```python
from build123d import *

# Parameters (mm, degrees)
F0_W = 76.971642673
F0_H = 95.2017754316


# Not quite as in the source:
# - a feature names something its author has since deleted; it is built from what else it names
# - the program builds the solid bodies; features that only make, move or delete a surface that nothing else refers to are left out


with BuildPart() as f2:
    # F2: sweep along a path in F1
    with BuildLine(Plane.XY) as f2_path:
        ThreePointArc((0, 0), (13.4369935077, -32.3954640503), (39.643291384, -55.703163147))
    # F0 (on Front) → F2 (sweep)
    with BuildSketch(Plane.XZ):
        Rectangle(F0_W, F0_H)
    sweep(path=f2_path.line)

    # F3: sweep along a path in F1
    with BuildLine(Plane.XY) as f3_path:
        ThreePointArc((-40.5113920569, -54.2563311756), (-14.8539477386, -31.1614707896), (0, 0))
    # F0 (on Front) → F3 (sweep)
    with BuildSketch(Plane.XZ):
        Rectangle(F0_W, F0_H)
    sweep(path=f3_path.line)


solid = f2.part
```
Model file for the job. Use its own axes, mm. A direction names the side the tool comes from. Coordinates: 2 decimals unless noted, no trailing zeros. Loops run counter-clockwise (first coordinate to the right, second up) from the corner with the lowest first, then second, coordinate; pieces in that order, holes last. Notation, with made-up numbers: M 7,-24 L 37,-24 A25 ccw 37,-4 Z; hole C -16,-35.5 d9. An arc over 180 degrees is marked long. Use CSV: the item, a comma, the result in double quotes. Start each with the question number.
1. Flat gauge pin, fed straight in: pin 1 (1.5 mm diameter, centred on y = -10.5, z = -1.5, fed in from +X). Where does the tip first touch, or does it go through?
2. Probe probe 1 along X at (y, z) = (-79, 15.5); probe 2 along X at (y, z) = (-77, -9); probe 3 along X at (y, z) = (-66, 1). List the from-to ranges inside material, lowest first. Write a range as [from, to].
3. Band-saw the part on B-B, the plane z = -1. List the corners of the cut face in (x, y).
4. Band-saw the part on C-C, the plane x = 5.5. List the corners of the cut face in (y, z), then the cut area to 3 significant figures.
5. Tool access for faces 1 (the cylindrical face through (47.899, -15.446, 0.666)), 2 (the cylindrical face through (6.5, -79.48, -0.67)): list every direction of +Z, -Z, +X, -X, +Y, -Y with a clear straight run to the whole face (end or side of a thin tool).
6. Two-plate mould, pull along X, no slides. Class faces 3 (the flat face through (1, 0, 1)), 4 (the flat face through (-40.892, -53.875, 0.666)), 5 (the cylindrical face through (-7.54, -77.19, 0.67)), 6 (the flat face through (39.309, -56.126, 0.666)): pulls with the +X half, pulls with the -X half, needs draft (parallel to the pull), parting line crosses it, or undercut.
7. Band-saw the part on A-A, the plane y = -74. List the corners of the cut face in (x, z).
8. Band-saw the part on D-D, the plane y = -38. List the corners of the cut face in (x, z), then the cut area to 3 significant figures.
Entries:
1,pin 1,"stops at x = 44.35"
2,probe 1,"x = [-15.81, -9.89], [5.88, 21.21]"
2,probe 2,"x = [-17.8, -7.3], [3.38, 22.79]"
2,probe 3,"x = [-28.79, 31.5]"
3,outline,"M -67.7,-27.02 L -13.32,-81.49 A126.05 ccw -1.87,-72.43 A116.6 ccw 15.76,-85.88 L 63.52,-25.52 A41.04 cw 38.49,0 L -38.49,0 A51.95 cw Z"
4,outline,"M -78.7,-47.6 L 0,-47.6 L 0,47.6 L -78.7,47.6 Z"
4,area,"7,490 mm2"
5,face 1,"+Z, -Z, +X, +Y"
5,face 2,"+Z, -Z, -Y"
6,face 3,"needs draft"
6,face 4,"pulls with the -X half"
6,face 5,"undercut"
6,face 6,"pulls with the +X half"
7,outline,"M -20.8,-47.6 L -3.67,-47.6 L -3.67,47.6 L -20.8,47.6 Z; M -0.13,-47.6 L 25.16,-47.6 L 25.16,47.6 L -0.13,47.6 Z"
8,outline,"M -56.74,-47.6 L 53.65,-47.6 L 53.65,47.6 L -56.74,47.6 Z"
8,area,"10,500 mm2"
